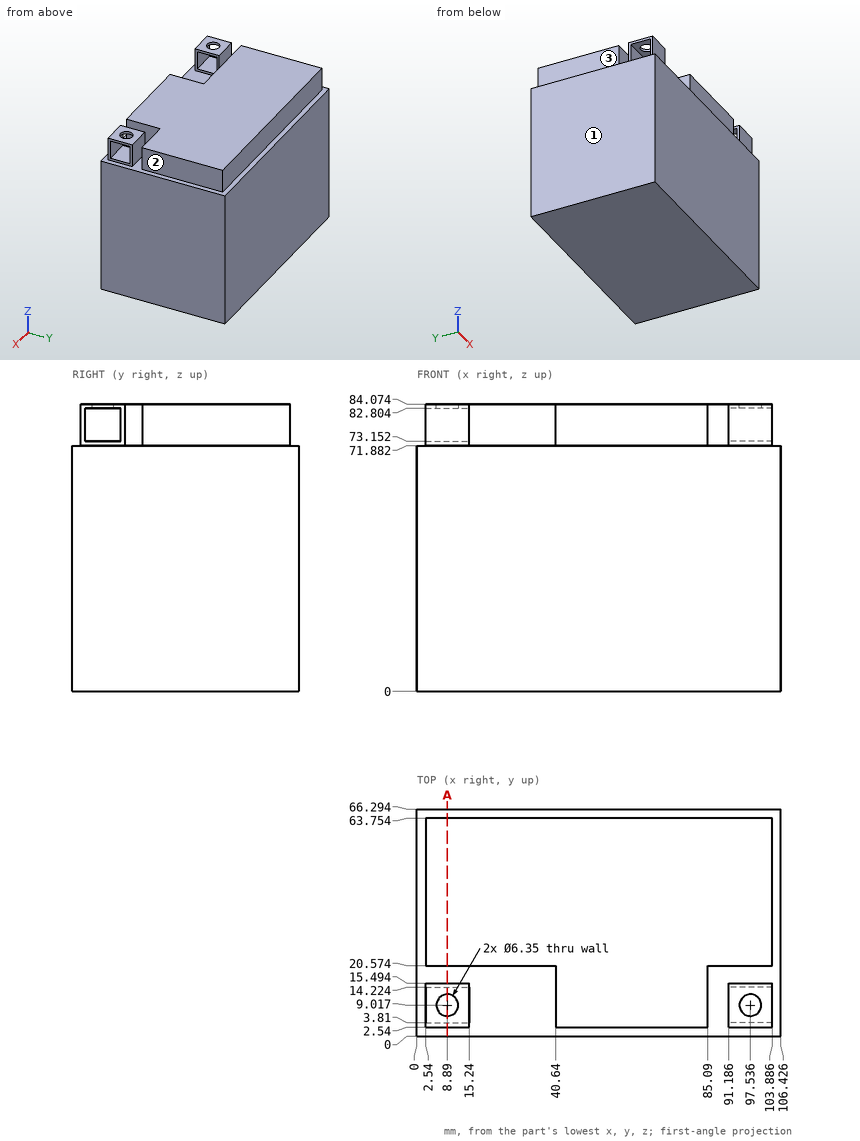
Check sheet for the drawn part. Datum: minimum x, y, z corner. Units: mm. A direction names the side the tool comes from. Give positions to 0.01 mm unless a question says otherwise; leave off trailing zeros. Loops run counter-clockwise (first coordinate to the right, second up) from the corner with the lowest first, then second, coordinate; pieces in that order, holes last. Notation, with made-up numbers: (6, 38.5) - (64, 38.5) arc R37 ccw to (64, 75.5) - close; hole circle Ø8 at (48.25, -12). An arc over 180 degrees is marked (long way). Write each question's results on one line, items separated by ' | '.
1) Sectioned sample at A-A on x = 8.89. Record the boundary of the cut face in (y, z).
Solution:
outline: (0, 0) - (66.29, 0) - (66.29, 71.88) - (63.75, 71.88) - (63.75, 84.07) - (20.57, 84.07) - (20.57, 71.88) - (15.49, 71.88) - (15.49, 84.07) - (12.19, 84.07) - (12.19, 82.8) - (14.22, 82.8) - (14.22, 73.15) - (3.81, 73.15) - (3.81, 82.8) - (5.84, 82.8) - (5.84, 84.07) - (2.54, 84.07) - (2.54, 71.88) - (0, 71.88) - close
2) Material ranges on L1, parallel to Y at x = 8, z = 83; L2, parallel to Z at x = 100, y = 4.5; L3, parallel to X at y = 54.5, z = 74, recorded low to high. Write a range as from..to.
Solution:
L1: 2.54..5.97, 12.06..15.49, 20.57..63.75 | L2: 0..73.15, 82.8..84.07 | L3: 2.54..103.89
3) Depth check by flat-ended pin: P1, Ø13.5, axis at y = 7, z = 76, coming from the +X side; P2, Ø3.5, axis at y = 9, z = 78, coming from the +X side; P3, Ø10, axis at y = 15, z = 81, coming from the -X side; P4, Ø5, axis at x = 6, z = 76.5, coming from the -Y side. Enter the tip coordinate at first touch or a pass-through.
Solution:
P1: x = 106.43 | P2: x = 85.09 | P3: x = 2.54 | P4: y = 2.54
4) Tool access check on the marked faces 1, 2 and 3. Record the directions out of +Z, -Z, +X, -X, +Y, -Y that give a thin tool (end or side, any length) a straight path to the whole face; none if there is none.
Solution:
face 1: +Z, -Z, -X, +Y, -Y | face 2: +Z, +X, +Y, -Y | face 3: +Z, -X, +Y, -Y
